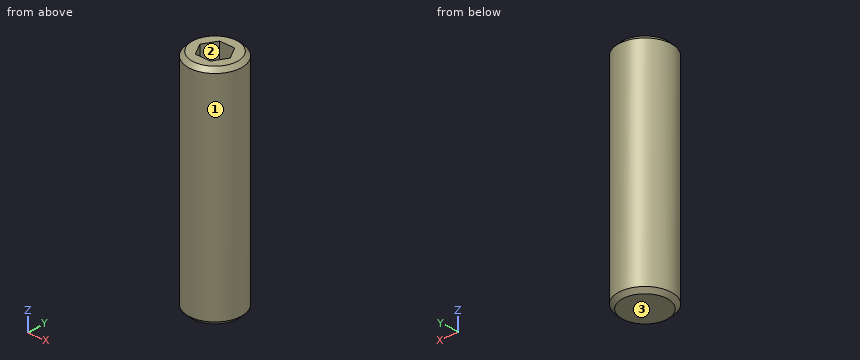
Solid Edge part; units mm, degrees
sketch "Sketch1" plane through (0, 0, 0) normal (0, 0, 1) x (1, 0, 0)
  circle A0 centre (0, 0) radius 3
extrude "Protrusion1" add sketch "Sketch1" along normal mid plane 25
chamfer "Chamfer1" distance 0.45 angle 45 2 edges at (-3, 0, -12.5) (-3, 0, 12.5)
sketch "Sketch2" plane through (0, 0, 12.5) normal (0, 0, 1) x (1, 0, 0)
  line L0 (-0.866, 1.5) -> (0.866, 1.5)
  line L1 (1.7321, 0) -> (0.866, 1.5)
  line L2 (0.866, -1.5) -> (1.7321, 0)
  line L3 (-0.866, -1.5) -> (0.866, -1.5)
  line L4 (-1.7321, 0) -> (-0.866, -1.5)
  line L5 (-0.866, 1.5) -> (-1.7321, 0)
extrude "Cutout1" cut sketch "Sketch2" against normal blind 12.5
properties part number "24104559"
Could you check a few things on this model? Use its own coordinates, in mm. Face numbers are marked on the shaded views. Give positions to 0.01 mm unless a question says otherwise; leave off trailing zeros. Write each loop counter-clockwise with the first axis right and the second up, starting at its lowest first coordinate (ties: lowest second). Pieces come first, ordered by that corner, then holes. Notation, with made-up numbers: (-2.75, 76.5) -> (33.25, 76.5) arc R26 cw to (33.25, 101.5) -> close; hole circle Ø8 at (-33.5, 74). An arc over 180 degrees is marked (long way). Answer as CSV lines item,"result". Start each with the question number.
(1) If we section it at C-C, the plane z = -7.5: Write out the boundary of the cut face in (x, y), and give its area (3 significant figures).
(2) If we section it at A-A, the plane z = 0.5: Write out the boundary of the cut face in (x, y).
(3) If we section it at B-B, the plane x = 0: Write out the boundary of the cut face in (y, z), and give its area (3 significant figures).
(4) I'm going to push flat-ended pins straight in: pin 1 Ø2.5 at (x, y) = (0, 0) entering from +Z; pin 2 Ø1 at (x, z) = (2, -8) entering from +Y; pin 3 Ø0.5 at (x, z) = (0.5, 8.5) entering from -Y. Where does each tip first touch, or does it pass through?
(5) Please list where these lines run through material, in increasing order: line 1 (Z direction, x = 0.3, y = 0.35); line 2 (X direction, y = -0.3, z = 4.5); line 3 (X direction, y = 0.65, z = 10.75).
(6) If we mould it in two halves opening along X, with no side actions, what happens to the marked faces 1, 2 and 3? For each: +X half, -X half, draft (parallel to the pull), parting line (faces both ways), or undercut.
Answer list:
1,outline,"circle Ø6 at (0, 0)"
1,area,"28.3 mm^2"
2,outline,"circle Ø6 at (0, 0); hole (-1.73, 0) -> (-0.87, -1.5) -> (0.87, -1.5) -> (1.73, 0) -> (0.87, 1.5) -> (-0.87, 1.5) -> close"
3,outline,"(-3, -12.05) -> (-2.55, -12.5) -> (2.55, -12.5) -> (3, -12.05) -> (3, 12.05) -> (2.55, 12.5) -> (1.5, 12.5) -> (1.5, 0) -> (-1.5, 0) -> (-1.5, 12.5) -> (-2.55, 12.5) -> (-3, 12.05) -> close"
3,area,"112 mm^2"
4,pin 1,"z = 0"
4,pin 2,"y = 2.6"
4,pin 3,"y = -2.99"
5,line 1,"-12.5 to 0"
5,line 2,"-2.98 to -1.56, 1.56 to 2.98"
5,line 3,"-2.93 to -1.36, 1.36 to 2.93"
6,face 1,"parting line"
6,face 2,"undercut"
6,face 3,"draft"
